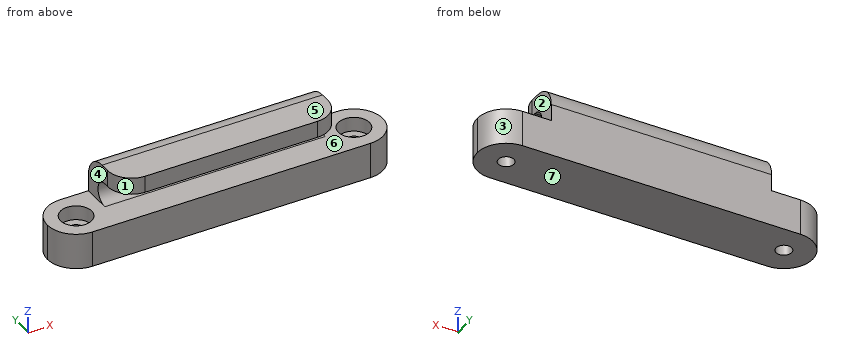
from build123d import *

# Parameters (mm, degrees)
SKETCH1_W           = 70
SKETCH1_H           = 12
BOSS_EXTRUDE1_DEPTH = 16
SKETCH2_R           = 2.5
CUT_EXTRUDE1_DEPTH  = 73.055534139
SKETCH3_W           = 5
SKETCH3_H           = 7.661898901
CUT_EXTRUDE2_DEPTH  = 73.055534139
SKETCH8_W           = 12
SKETCH8_H           = 12
CUT_EXTRUDE6_DEPTH  = 8.5
FILLET2_R           = 5
SKETCH9_R           = 1.625
CUT_EXTRUDE7_DEPTH  = 37.513696061
SKETCH10_R          = 3.25
CUT_EXTRUDE8_DEPTH  = 3
FILLET3_R           = 6
FILLET5_R           = 5


with BuildPart() as part:
    # Sketch1 → Boss-Extrude1 (new body)
    with BuildSketch(Plane.XY):
        Rectangle(SKETCH1_W, SKETCH1_H)
    extrude(amount=BOSS_EXTRUDE1_DEPTH)

    # Sketch2 → Cut-Extrude1 (cut, through all)
    with BuildSketch(Plane.ZY.offset(35)):
        with Locations((10, 0)):
            Circle(SKETCH2_R)
    extrude(amount=-CUT_EXTRUDE1_DEPTH, mode=Mode.SUBTRACT)

    # Sketch3 → Cut-Extrude2 (cut, through all)
    with BuildSketch(Plane.ZY.offset(35)):
        with Locations((10, -3.830949451)):
            Rectangle(SKETCH3_W, SKETCH3_H)
    extrude(amount=-CUT_EXTRUDE2_DEPTH, mode=Mode.SUBTRACT)

    # Sketch8 → Cut-Extrude6 (cut)
    with BuildSketch(Plane.XY.offset(16)):
        with Locations((-29, 0)):
            Rectangle(SKETCH8_W, SKETCH8_H)
        with Locations((29, 0)):
            Rectangle(SKETCH8_W, SKETCH8_H)
    extrude(amount=-CUT_EXTRUDE6_DEPTH, mode=Mode.SUBTRACT)

    # Fillet2
    fillet2_edges = [part.edges().sort_by_distance(p)[0] for p in [
        (0, 6, 16),
    ]]
    fillet(fillet2_edges, radius=FILLET2_R)

    # Sketch9 → Cut-Extrude7 (cut, through all)
    with BuildSketch(Plane.XY.offset(7.5)):
        with Locations((-29, 0)):
            Circle(SKETCH9_R)
        with Locations(Location((29, 0, 0), (0, 0, 180))):
            Circle(SKETCH9_R)
    extrude(amount=-CUT_EXTRUDE7_DEPTH, mode=Mode.SUBTRACT)

    # Sketch10 → Cut-Extrude8 (cut)
    with BuildSketch(Plane.XY.offset(7.5)):
        with Locations((-29, 0)):
            Circle(SKETCH10_R)
        with Locations(Location((29, 0, 0), (0, 0, 180))):
            Circle(SKETCH10_R)
    extrude(amount=-CUT_EXTRUDE8_DEPTH, mode=Mode.SUBTRACT)

    # Fillet3
    fillet3_edges = [part.edges().sort_by_distance(p)[0] for p in [
        (35, 6, 3.75),
        (35, -6, 3.75),
        (-35, 6, 3.75),
        (-35, -6, 3.75),
    ]]
    fillet(fillet3_edges, radius=FILLET3_R - 0.0001)  # a hair under: the kernel refuses the full size

    # Fillet5
    fillet5_edges = [part.edges().sort_by_distance(p)[0] for p in [
        (-23, -6, 14.25),
        (23, -6, 14.25),
    ]]
    fillet(fillet5_edges, radius=FILLET5_R)


solid = part.part
Part model, mm, in its own coordinate system. Face numbers are marked on the shaded views. A direction names the side the tool comes from. Give positions to 0.01 mm unless a question says otherwise; leave off trailing zeros. Loops run counter-clockwise (first coordinate to the right, second up) from the corner with the lowest first, then second, coordinate; pieces in that order, holes last.
(1) Drill centre lines: line 1 along Z through (x, y) = (16.5, -2); line 2 along Y through (x, z) = (-29, 6.4); line 3 along Y through (x, z) = (-29, 2.9) (3 decimals). Where is each one in solid material? Low to high.
Return value:
line 1: z = 0 to 7.5, 12.5 to 16
line 2: y = -6 to -3.25, 3.25 to 6
line 3: y = -6 to -1.625, 1.625 to 6
(2) Band-saw the part on A-A (z = 6.75). Count the separate pieces of the cut face and the enclosed holes in it, and give its area (3 significant figures).
Return value:
separate pieces: 1
enclosed holes: 2
area: 743 mm2
(3) Band-saw the part on B-B (x = 22). Write the cut outline in (y, z).
Return value:
outline: (-6, 0) - (6, 0) - (6, 11) arc R5 ccw to (1, 16) - (-4, 16) - (-4, 12.5) - (0, 12.5) arc R2.5 cw to (0, 7.5) - (-6, 7.5) - close
(4) 3-axis set-ups, long thin cutter, end or side, ignore diameter. For the marked faces 1, 2 and 3: which of +Z, -Z, +X, -X, +Y, -Y reach the whole face in a straight line?
Return value:
face 1: +Z, -X, -Y
face 2: +Z, +X, +Y, -Y
face 3: +Z, -Z, +X, +Y
(5) Band-saw the part on C-C (z = 14). Write the cut outline in (x, y).
Return value:
outline: (-23, -1) arc R5 ccw to (-18, -6) - (18, -6) arc R5 ccw to (23, -1) - (23, 5) - (-23, 5) - close
(6) Band-saw the part on D-D (x = 6). Write the cut outline in (y, z), and give its area (3 significant figures).
Return value:
outline: (-6, 0) - (6, 0) - (6, 11) arc R5 ccw to (1, 16) - (-6, 16) - (-6, 12.5) - (0, 12.5) arc R2.5 cw to (0, 7.5) - (-6, 7.5) - close
area: 147 mm2
(7) Pull direction Z, two halves, no side cores. Call the marked faces 4, 5, 6 and 7: pulls with the +Z half, pulls with the -Z half, needs draft (parallel to the pull), parting line crosses it, or undercut.
Return value:
face 4: needs draft
face 5: pulls with the +Z half
face 6: undercut
face 7: pulls with the -Z half
(8) Pin check, flat tips, straight feed: pin 1 (1.5 mm diameter, centred on y = 2.5, z = 8, fed in from +X); pin 2 (5 mm diameter, centred on x = 29, y = 0, fed in from +Z); pin 3 (5.5 mm diameter, centred on y = 3.5, z = 10, fed in from +X); pin 4 (2.5 mm diameter, centred on x = -29, y = 0, fed in from +Z). Stop position of each tip, or through.
Return value:
pin 1: stops at x = 34.68
pin 2: stops at z = 4.5
pin 3: stops at x = 34.52
pin 4: passes through
